The drawing under review shows one solid part. Ordinate dimensions are in mm from its lowest x, y, z. Give positions to 0.01 mm unless a question says otherwise; leave off trailing zeros. Write each loop counter-clockwise with the first axis right and the second up, starting at its lowest first coordinate (ties: lowest second). Pieces come first, ordered by that corner, then holes. Notation, with made-up numbers: (-39, 4) -> (13, 4) arc R32 cw to (13, 30) -> close; hole circle Ø3 at (-28.75, -18.75). An arc over 180 degrees is marked (long way). Answer as a JSON object with one key per item and string values.
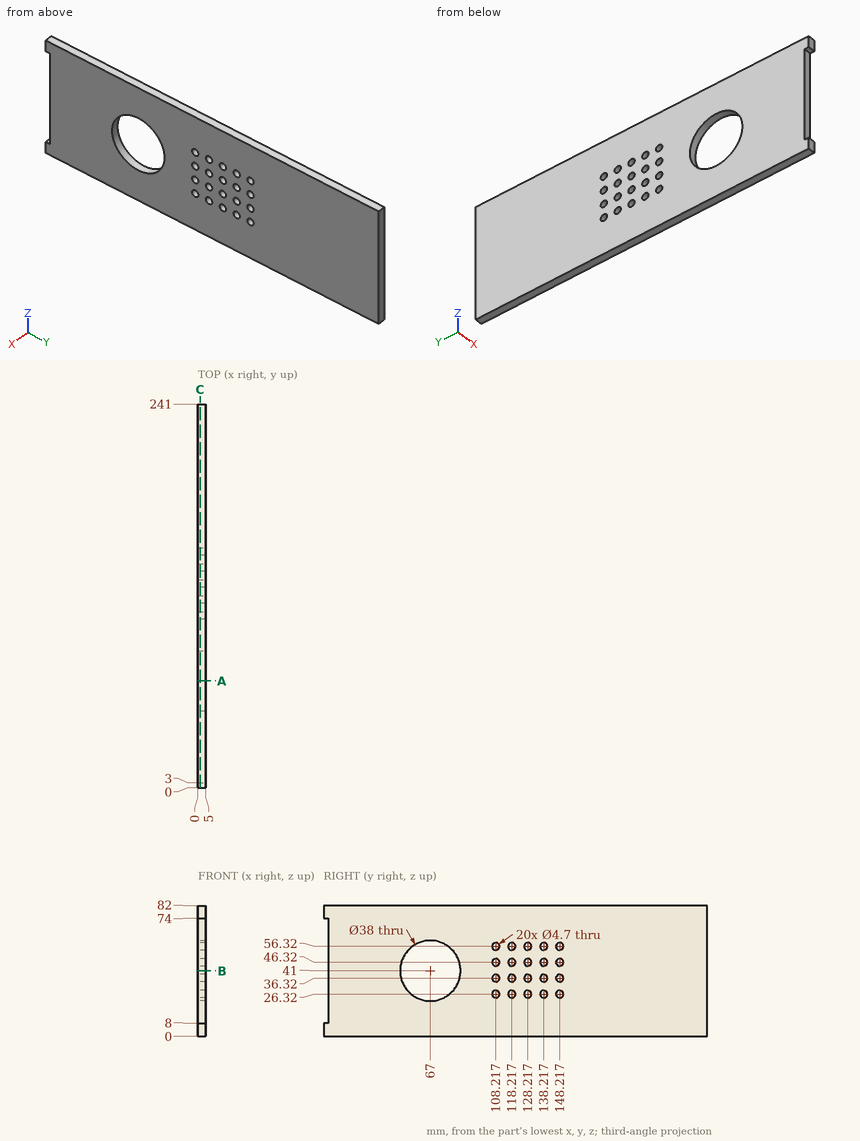
(1) We need section B-B, the plane z = 41. State the section outline as (x, y) points, then the cut area to 3 significant figures.
Here are the results:
{"outline": "(0, 3) -> (5, 3) -> (5, 48) -> (0, 48) -> close; (0, 86) -> (5, 86) -> (5, 241) -> (0, 241) -> close", "area": "1,000 mm²"}
(2) Clearance check with flat-ended pins moving along their axes: pin 1 (4 mm diameter, centred on y = 136.5, z = 40.5, fed in from -X); pin 2 (3 mm diameter, centred on y = 148.22, z = 26.32, fed in from +X); pin 3 (2 mm diameter, centred on x = 4, z = 17, fed in from -Y). State where each tip first meets the part, or that it passes through.
Here are the results:
{"pin 1": "stops at x = 0", "pin 2": "passes through", "pin 3": "stops at y = 3"}
(3) We need section A-A, the plane y = 67. State the section outline as (x, z) points, then the cut area to 3 significant figures.
Here are the results:
{"outline": "(0, 0) -> (5, 0) -> (5, 22) -> (0, 22) -> close; (0, 60) -> (5, 60) -> (5, 82) -> (0, 82) -> close", "area": "220 mm²"}
(4) We need section C-C, the plane x = 1.45. Give the number of separate pieces and of enclosed holes in the cut face, then the cut area to 3 significant figures.
Here are the results:
{"separate pieces": "1", "enclosed holes": "21", "area": "18,100 mm²"}
(5) For line 1 along Z through (x, y) = (2, 116.5) (1 decimal); line 2 along Y through (x, z) = (0.7, 42); line 3 along Y through (x, z) = (3, 70.5), list the stretches that pass through material, from the lowest coordinate up.
Here are the results:
{"line 1": "z = 0 to 24.7, 27.9 to 34.7, 37.9 to 44.7, 47.9 to 54.7, 57.9 to 82", "line 2": "y = 3 to 48.03, 85.97 to 241", "line 3": "y = 3 to 241"}
